Autodesk Inventor part; units mm, degrees
ref_plane "YZ Plane" through (0, 0, 0) normal (1, 0, 0) x (0, 1, 0)
ref_plane "XZ Plane" through (0, 0, 0) normal (0, 1, 0) x (-1, 0, 0)
ref_plane "XY Plane" through (0, 0, 0) normal (0, 0, 1) x (1, 0, 0)
sketch "Sketch1" plane through (0, 0, 0) normal (0, 0, 1) x (1, 0, 0)
  line L0 (-12.1708, 16.0073) -> (13.2292, 16.0073)
  line L1 (13.2292, 16.0073) -> (13.2292, -34.7927)
  line L2 (13.2292, -34.7927) -> (-12.1708, -34.7927)
  line L3 (-12.1708, -34.7927) -> (-12.1708, 16.0073)
  line L4 (11.9592, 14.7373) -> (-10.9008, 14.7373)
  line L5 (-10.9008, 14.7373) -> (-10.9008, -33.5227)
  line L6 (-10.9008, -33.5227) -> (11.9592, -33.5227)
  line L7 (11.9592, -33.5227) -> (11.9592, 14.7373)
  point P0 (0, 0)
  dimension "d0" = 25.4
  dimension "d1" = 50.8
  dimension "d2" = 1.27
extrude "Extrusion1" add sketch "Sketch1" along normal blind 254
sketch "Sketch2" plane through (-12.1708, 16.0073, 0) normal (0, 1, 0) x (1, 0, 0)
  circle A0 centre (12.7, -12.7) radius 1.7272
  line L0 (25.4, 0) -> (0, 0)
  line L1 (0, 0) -> (0, -254)
  point P0 (12.1708, 0)
  dimension "d5" = 3.4544
  dimension "d6" = 12.7
  dimension "d7" = 12.7
extrude "Extrusion2" cut sketch "Sketch2" against normal through all
pattern_linear "Rectangular Pattern1" count 10 spacing 25.4 along (0, 0, 1) of "Extrusion2"
equation "\"d3\" = d13"
equation "\"d13\" = 254"
properties part number "VerseFrame 10in"
The listing builds one solid part. Answer for the finished solid, in the listing's coordinates (mm). A direction names the side the tool comes from. Coordinates: 2 decimals unless noted, no trailing zeros. Loops run counter-clockwise (first coordinate to the right, second up) from the corner with the lowest first, then second, coordinate; pieces in that order, holes last. Notation, with made-up numbers: (-18.5, 34) -> (-8.5, 34) arc R17 ccw to (-8.5, 51) -> close; hole circle Ø8 at (86.5, 3.25). An arc over 180 degrees is marked (long way). Answer in a Markdown table with one row per item. Add a question column.
1. The part is cut by section C-C, the plane z = 94. Write down the section's boundary in (x, y), then the cut area to 3 significant figures.
2. The part is cut by section A-A, the plane x = -6.25. Write down the section's boundary in (y, z), then the cut area to 3 significant figures.
3. Determine the mould class of faces 3 (the flat face through (13.229, -9, 125)), 4 (the flat face through (1, 14.737, 125)), 5 (the flat face through (-10.901, -9, 125)), 6 (the flat face through (0, 16.007, 125)) for opening direction Y: +Y half, -Y half, draft (parallel to the pull), parting line (faces both ways), or undercut.
4. Consider line 1 (Y direction, x = -0.5, z = 151); line 2 (X direction, y = 13, z = 92); line 3 (X direction, y = 15, z = 114). Determine where each line is inside the solid, lowest interval first. Write a range as [from, to].
5. For faces 1 (the flat face through (-12.171, -10, 125)), 2 (the flat face through (11.959, -10, 125)), determine the directions among +Z, -Z, +X, -X, +Y, -Y from which every point of the face is accessible in a straight line to the end or side of a thin tool.
6. The part is cut by section B-B, the plane y = -13. Write down the section's boundary in (x, z), then the cut area to 3 significant figures.
Answer below:
| question | item | result |
|---|---|---|
| 1 | outline | (-12.17, -34.79) -> (13.23, -34.79) -> (13.23, 16.01) -> (-12.17, 16.01) -> close; hole (-10.9, -33.52) -> (11.96, -33.52) -> (11.96, 14.74) -> (-10.9, 14.74) -> close |
| 1 | area | 187 mm2 |
| 2 | outline | (-34.79, 0) -> (-33.52, 0) -> (-33.52, 254) -> (-34.79, 254) -> close; (14.74, 0) -> (16.01, 0) -> (16.01, 254) -> (14.74, 254) -> close |
| 2 | area | 645 mm2 |
| 3 | face 3 | draft |
| 3 | face 4 | undercut |
| 3 | face 5 | undercut |
| 3 | face 6 | +Y half |
| 4 | line 1 | [-34.79, -33.52], [14.74, 16.01] |
| 4 | line 2 | [-12.17, -10.9], [11.96, 13.23] |
| 4 | line 3 | [-12.17, -1.17], [2.23, 13.23] |
| 5 | face 1 | +Z, -Z, -X, +Y, -Y |
| 5 | face 2 | +Z, -Z |
| 6 | outline | (-12.17, 0) -> (-10.9, 0) -> (-10.9, 254) -> (-12.17, 254) -> close; (11.96, 0) -> (13.23, 0) -> (13.23, 254) -> (11.96, 254) -> close |
| 6 | area | 645 mm2 |
